Verification items for the finished model (mm, model axes). Face numbers are marked on the shaded views. A direction names the side the tool comes from. Give positions to 0.01 mm unless a question says otherwise; leave off trailing zeros. Loops run counter-clockwise (first coordinate to the right, second up) from the corner with the lowest first, then second, coordinate; pieces in that order, holes last. Notation, with made-up numbers: M -14,19.25 L 17,19.25 A31 ccw 17,48.25 Z; hole C -37,88.5 d10. An arc over 180 degrees is marked long. Answer in a Markdown table with one row per item.
```python
from build123d import *

# Parameters (mm, degrees)
DODANIE_WYCI_GNI_CIE1_DEPTH = 4
ZAOKR_GLENIE1_R             = 1.8
SZKIC2_W                    = 4
SZKIC2_H                    = 6
DODANIE_WYCI_GNI_CIE2_DEPTH = 3
ZAOKR_GLENIE2_R             = 2
SZKIC3_W                    = 4
SZKIC3_H                    = 12
DODANIE_WYCI_GNI_CIE3_DEPTH = 4
SFAZOWANIE1_SIZE            = 2.5


with BuildPart() as part:
    # Szkic1 → Dodanie-wyciągnięcie1 (new body)
    with BuildSketch(Plane.XY):
        Polygon((0, 0), (0, 25), (2, 25), (2, 3), (3.5, 3), (3.5, 23), (2.5, 23), (2.5, 25), (5, 25), (5, 0), align=None)
    extrude(amount=DODANIE_WYCI_GNI_CIE1_DEPTH)

    # Zaokrąglenie1
    zaokr_glenie1_edges = [part.edges().sort_by_distance(p)[0] for p in [
        (5, 25, 2),
        (5, 0, 2),
    ]]
    fillet(zaokr_glenie1_edges, radius=ZAOKR_GLENIE1_R)

    # Szkic2 → Dodanie-wyciągnięcie2 (add)
    with BuildSketch(Plane.ZY):
        with Locations((2, 12.5)):
            Rectangle(SZKIC2_W, SZKIC2_H)
    extrude(amount=DODANIE_WYCI_GNI_CIE2_DEPTH)

    # Zaokrąglenie2
    zaokr_glenie2_edges = [part.edges().sort_by_distance(p)[0] for p in [
        (-1.5, 15.5, 0),
        (-1.5, 9.5, 4),
    ]]
    fillet(zaokr_glenie2_edges, radius=ZAOKR_GLENIE2_R)

    # Szkic3 → Dodanie-wyciągnięcie3 (add)
    with BuildSketch(Plane.ZY.offset(3)):
        with Locations((2, 12.5)):
            Rectangle(SZKIC3_W, SZKIC3_H)
    extrude(amount=DODANIE_WYCI_GNI_CIE3_DEPTH)

    # Sfazowanie1
    sfazowanie1_edges = [part.edges().sort_by_distance(p)[0] for p in [
        (-7, 6.5, 2),
        (-7, 18.5, 2),
    ]]
    chamfer(sfazowanie1_edges, length=SFAZOWANIE1_SIZE)


solid = part.part
```
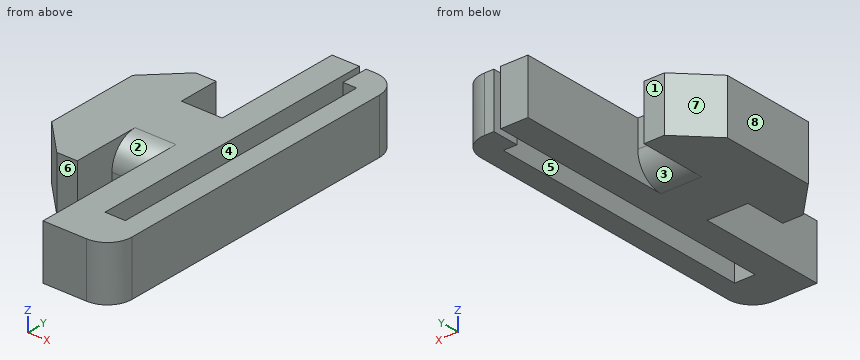
Item 1: Sectioned sample at B-B (y = 7). Record the cut outline in (x, z), and give its area (3 significant figures).
Reported:
| item | result |
|---|---|
| outline | M -5,0 L -3,0 L -3,4 L -5,4 Z; M 0,0 L 2,0 L 2,4 L 0,4 Z; M 3.5,0 L 5,0 L 5,4 L 3.5,4 Z |
| area | 22.0 mm^2 |
Item 2: Sectioned sample at A-A (y = 11.75). Record the cut outline in (x, z).
Reported:
| item | result |
|---|---|
| outline | M -7,0 L 2,0 L 2,4 L -7,4 Z; M 3.5,0 L 5,0 L 5,4 L 3.5,4 Z |
Item 3: Scan lines: L1, parallel to X at y = 15.25, z = 0.4; L2, parallel to X at y = 4.5, z = 3.7; L3, parallel to X at y = 13.5, z = 1.3. Record each from-to range of solid material in increasing order. Write a range as [from, to].
Reported:
| item | result |
|---|---|
| L1 | x = [-7, -3], [0, 2], [3.5, 5] |
| L2 | x = [0, 2], [3.5, 5] |
| L3 | x = [-7, 2], [3.5, 5] |
Item 4: Release check for a two-part mould opening along Y. For the marked faces 5, 6, 7 and 8 record: released by +Y, released by -Y, zero draft, split by the parting line, or undercut.
Reported:
| item | result |
|---|---|
| face 5 | undercut |
| face 6 | released by -Y |
| face 7 | released by +Y |
| face 8 | zero draft |
Item 5: Sectioned sample at D-D (x = -1.5). Record the cut outline in (y, z).
Reported:
| item | result |
|---|---|
| outline | M 9.5,0 L 13.5,0 A2 ccw 15.5,2 L 15.5,4 L 11.5,4 A2 ccw 9.5,2 Z |
Item 6: Tool access check on the marked faces 1, 2, 3 and 4. Record the directions out of +Z, -Z, +X, -X, +Y, -Y that give a thin tool (end or side, any length) a straight path to the whole face; none if there is none.
Reported:
| item | result |
|---|---|
| face 1 | +Z, -Z, -X, +Y |
| face 2 | +Z, -Y |
| face 3 | -Z, +Y |
| face 4 | +Z, -Z, +Y |
Item 7: Go/stop test with flat-tipped pins: pin 1 (1.2 mm diameter, centred on y = 7.5, z = 2.5, fed in from -X); pin 2 (1 mm diameter, centred on x = -1, z = 1, fed in from -Y); pin 3 (0.5 mm diameter, centred on x = -3.5, z = 2.5, fed in from +Y). Record where each tip stops, or that it passes through.
Reported:
| item | result |
|---|---|
| pin 1 | stops at x = -6.1 |
| pin 2 | stops at y = 9.5 |
| pin 3 | stops at y = 18.5 |
Item 8: Sectioned sample at C-C (z = 3.6). Record the cut outline in (x, y).
Reported:
| item | result |
|---|---|
| outline | M -7,9 L -4.5,6.5 L -3,6.5 L -3,10.3 L 0,10.3 L 0,0 L 3.2,0 A1.8 ccw 5,1.8 L 5,23.2 A1.8 ccw 3.2,25 L 2.5,25 L 2.5,23 L 3.5,23 L 3.5,3 L 2,3 L 2,25 L 0,25 L 0,15.5 L -3,15.5 L -3,18.5 L -4.5,18.5 L -7,16 Z |
